Model file for the job. Use its own axes, mm. A direction names the side the tool comes from. Round coordinates to 2 decimals unless told otherwise and drop trailing zeros. Order: outer loops, then holes, each group sorted by start corner. A loop starts at its lowest first (then second) coordinate and runs counter-clockwise, first axis right, second up. Notation, with made-up numbers: (21, 75) -> (67, 75) arc R35 ccw to (67, 114) -> close; hole circle Ø4 at (65, -23.75). An arc over 180 degrees is marked (long way). Put each result on its own line as item: value. Start each with the question number.
Q1. Probe L1, parallel to X at y = 76, z = 0; L2, parallel to X at y = 0.75, z = 0; L3, parallel to Y at x = -8.5, z = 14. List the from-to ranges inside material, lowest first.
Q2. Flat gauge pins, fed straight in: P1, Ø1.5, axis at x = -5, y = 59.5, coming from the -Z side; P2, Ø2, axis at y = 20, z = 10.5, coming from the -X side; P3, Ø1.5, axis at y = 35.5, z = -10.5, coming from the +X side; P4, Ø6, axis at y = 62, z = -15, coming from the +X side. Where does each tip first touch, or does it go through?
Q3. Cut at C-C, the plane y = 27.5. List the corners of the cut face in (x, z).
Q4. Cut at A-A, the plane z = 17. List the corners of the cut face in (x, y), and give its area (3 significant figures).
Q5. 3-axis set-ups, long thin cutter, end or side, ignore diameter. For faces 1 (the face through (0, 1, 0)), 2 (the face through (-3.905, 76.035, -0.867)), 3 (the face through (10.5, 77.99, 6.78)): which of +Z, -Z, +X, -X, +Y, -Y reach the whole face in a straight line?
Q6. Cut at D-D, the plane y = 72. List the corners of the cut face in (x, z).
Q7. Cut at B-B, the plane x = 19. List the corners of the cut face in (y, z) (3 decimals).
from build123d import *

# Parameters (mm, degrees)
SKETCH1_R           = 20
BOSS_EXTRUDE1_DEPTH = 50.5
SKETCH2_R           = 21.5
BOSS_EXTRUDE2_DEPTH = 7
BOSS_EXTRUDE3_DEPTH = 1
SKETCH5_R           = 5
CUT_EXTRUDE1_DEPTH  = 1
SKETCH6_R           = 4
CUT_EXTRUDE2_DEPTH  = 5


with BuildPart() as part:
    # Sketch1 → Boss-Extrude1 (new body)
    with BuildSketch(Plane(origin=(0, 0, 0), x_dir=(1, 0, 0), z_dir=(0, 1, 0))):
        with Locations(Location((0, 0, 0), (0, 0, 270))):
            Circle(SKETCH1_R)
    extrude(amount=BOSS_EXTRUDE1_DEPTH)

    # Sketch2 → Boss-Extrude2 (add)
    with BuildSketch(Plane(origin=(0, 50.5, 0), x_dir=(1, 0, 0), z_dir=(0, 1, 0))):
        with Locations(Location((0, 0, 0), (0, 0, 270))):
            Circle(SKETCH2_R)
    extrude(amount=BOSS_EXTRUDE2_DEPTH)

    # Sketch3 → Revolve1 (revolve)
    with BuildSketch(Plane.XY, mode=Mode.PRIVATE) as revolve1_sk:
        with BuildLine():
            Line((0, 77.5), (12.5, 77.5))
            ThreePointArc((12.5, 77.5), (9.674701278, 67.5), (12.5, 57.5))
            Line((12.5, 57.5), (0, 57.5))
            Line((0, 57.5), (0, 77.5))
        make_face()
    revolve(revolve1_sk.sketch.rotate(Axis((0, 57.5, 0), (0, 1, 0)), 90), axis=Axis((0, 57.5, 0), (0, 1, 0)))

    # Sketch4 → Boss-Extrude3 (add)
    with BuildSketch(Plane(origin=(0, 77.5, 0), x_dir=(1, 0, 0), z_dir=(0, 1, 0))):
        Polygon((8.841834545, 9.179007009), (4.656136058, 11.863920297), (-0.238416936, 12.742659266), (-5.096673112, 11.681443874), (-9.179007009, 8.841834545), (-11.863920297, 4.656136058), (-12.742659266, -0.238416936), (-11.681443874, -5.096673112), (-8.841834545, -9.179007009), (-4.656136058, -11.863920297), (0.238416936, -12.742659266), (5.096673112, -11.681443874), (9.179007009, -8.841834545), (11.863920297, -4.656136058), (12.742659266, 0.238416936), (11.681443874, 5.096673112), align=None)
    extrude(amount=BOSS_EXTRUDE3_DEPTH)

    # Sketch5 → Cut-Extrude1 (cut)
    with BuildSketch(Plane.XZ):
        with Locations(Location((0, 0, 0), (0, 0, 270))):
            Circle(SKETCH5_R)
    extrude(amount=-CUT_EXTRUDE1_DEPTH, mode=Mode.SUBTRACT)

    # Sketch6 → Cut-Extrude2 (cut)
    with BuildSketch(Plane(origin=(0, 78.5, 0), x_dir=(1, 0, 0), z_dir=(0, 1, 0))):
        with Locations(Location((0, 0, 0), (0, 0, 270))):
            Circle(SKETCH6_R)
    extrude(amount=-CUT_EXTRUDE2_DEPTH, mode=Mode.SUBTRACT)


solid = part.part
Ans:
1. L1: x = -11.67 to -4, 4 to 11.67
1. L2: x = -20 to -5, 5 to 20
1. L3: y = 0 to 57.5
2. P1: stops at z = -10.8
2. P2: stops at x = -17.6
2. P3: stops at x = 17.46
2. P4: passes through
3. outline: circle Ø40 at (0, 0)
4. outline: (-13.16, 50.5) -> (-10.54, 50.5) -> (-10.54, 0) -> (10.54, 0) -> (10.54, 50.5) -> (13.16, 50.5) -> (13.16, 57.5) -> (-13.16, 57.5) -> close
4. area: 1,250 mm^2
5. face 1: -Y
5. face 2: +Y
5. face 3: +Z, +X, +Y
6. outline: circle Ø20.42 at (0, 0)
7. outline: (0, -6.245) -> (50.5, -6.245) -> (50.5, -10.062) -> (57.5, -10.062) -> (57.5, 10.062) -> (50.5, 10.062) -> (50.5, 6.245) -> (0, 6.245) -> close
